Geometry check sheet. Reference: the model listing, model coordinates, mm. A direction names the side the tool comes from. Coordinates: 2 decimals unless noted, no trailing zeros. Loops run counter-clockwise (first coordinate to the right, second up) from the corner with the lowest first, then second, coordinate; pieces in that order, holes last.
from build123d import *

# Parameters (mm, degrees)
SKETCH1_R           = 1.617686351
BOSS_EXTRUDE1_DEPTH = 3.175
CUT_EXTRUDE1_DEPTH  = 1.5875


with BuildPart() as part:
    # Sketch1 → Boss-Extrude1 (new body)
    with BuildSketch(Plane.XY):
        with BuildLine():
            Line((2.376512113, 27.65079512), (87.842998078, 27.65079512))
            ThreePointArc((87.842998078, 27.65079512), (95.027202975, 24.675000017), (98.002998078, 17.49079512))
            Line((98.002998078, 17.49079512), (98.002998078, 7.726780525))
            ThreePointArc((98.002998078, 7.726780525), (95.027202975, 0.542575628), (87.842998078, -2.433219475))
            Line((87.842998078, -2.433219475), (2.376512113, -2.433219475))
            ThreePointArc((2.376512113, -2.433219475), (-4.807692784, 0.542575628), (-7.783487887, 7.726780525))
            Line((-7.783487887, 7.726780525), (-7.783487887, 17.49079512))
            ThreePointArc((-7.783487887, 17.49079512), (-4.807692784, 24.675000017), (2.376512113, 27.65079512))
        make_face()
        with Locations((-4.068268159, 12.608787822)):
            Circle(SKETCH1_R, mode=Mode.SUBTRACT)
    extrude(amount=BOSS_EXTRUDE1_DEPTH)

    # Sketch2 → Cut-Extrude1 (cut)
    # profile 1 of 3: a face of its own
    with BuildSketch(Plane.XY.offset(3.175)):
        with BuildLine():
            add(Edge.make_bspline(
                [(26.055314757, 25.363302374), (26.281041178, 25.357148606), (26.720344033, 25.345172305), (27.358603179, 25.255576736), (27.954181106, 25.10565776), (28.506593472, 24.887414053), (29.01635882, 24.61026015), (29.483989025, 24.268912351), (29.909556765, 23.870244327), (30.286214231, 23.412653315), (30.607890769, 22.914633219), (30.869796512, 22.384371241), (31.05896534, 21.825349006), (31.177064683, 21.240476881), (31.238829311, 20.630578255), (31.216595671, 19.996303633), (31.140690223, 19.333888525), (31.036825384, 18.891448023), (30.983281734, 18.663364293)],
                knots=[0, 0, 0, 0, 1.104647112, 2.14983532, 3.14775057, 4.103991838, 5.04949864, 5.980264506, 6.930364641, 7.896350518, 8.873894228, 9.826455567, 10.784034957, 11.753687545, 12.741876869, 13.777217861, 14.854127416, 16, 16, 16, 16], degree=3))
            Line((30.983281734, 18.663364293), (24.823323013, 14.893993808))
            add(Edge.make_bspline(
                [(24.823323013, 14.893993808), (24.913627964, 14.852436986), (25.056727556, 14.786584956), (25.204086092, 14.731009487), (25.258452012, 14.710505676)],
                knots=[0, 0, 0, 0, 1.262127295, 2, 2, 2, 2], degree=3))
            add(Edge.make_bspline(
                [(25.258452012, 14.710505676), (25.408658011, 14.633015541), (25.70455598, 14.480364025), (26.115294044, 14.203511612), (26.494533839, 13.898795938), (26.842207753, 13.563435468), (27.152694985, 13.192982522), (27.431219321, 12.792771569), (27.67927879, 12.362334709), (27.886089668, 11.901078686), (28.060682724, 11.422012006), (28.186061, 10.924600148), (28.269482345, 10.415995768), (28.312768514, 9.893514579), (28.306836135, 9.356553203), (28.251637963, 8.806740636), (28.160254496, 8.243184587), (28.061167889, 7.870056205), (28.010773994, 7.680288958)],
                knots=[0, 0, 0, 0, 0.984435104, 1.939285714, 2.881007598, 3.817426453, 4.749903878, 5.693661681, 6.656357472, 7.640950646, 8.636494269, 9.624663586, 10.626026113, 11.637696297, 12.67668649, 13.751023199, 14.856205644, 16, 16, 16, 16], degree=3))
            add(Edge.make_bspline(
                [(28.010773994, 7.680288958), (27.934336699, 7.418635325), (27.781985703, 6.897120378), (27.483880814, 6.140182715), (27.111873403, 5.418274722), (26.680602198, 4.723985098), (26.188457087, 4.059016869), (25.632410614, 3.42464569), (25.013362966, 2.8218799), (24.336555177, 2.259555831), (23.632617641, 1.73501911), (22.90194296, 1.286167719), (22.165575056, 0.899844078), (21.419750266, 0.582322921), (20.662474561, 0.341850589), (19.896429331, 0.167011128), (19.120780451, 0.059173369), (18.599040207, 0.044186513), (18.338328173, 0.036697626)],
                knots=[0, 0, 0, 0, 0.992207688, 1.977618791, 2.956517026, 3.945270844, 4.9506118, 5.965172583, 7.01356654, 8.093011568, 9.167098768, 10.207118156, 11.211733991, 12.192594754, 13.154449955, 14.10064625, 15.050898635, 16, 16, 16, 16], degree=3))
            Line((18.338328173, 0.036697626), (-1.667120743, 0.036697626))
            Line((-1.667120743, 0.036697626), (5.148152735, 25.363302374))
            Line((5.148152735, 25.363302374), (26.055314757, 25.363302374))
        make_face()
        Polygon((20.472033024, 6.196656347), (22.396037152, 13.373663571), (16.304231166, 9.567595459), (10.872982456, 9.567595459), (7.428648091, 6.196656347), align=None, mode=Mode.SUBTRACT)
        Polygon((22.867863777, 15.108937049), (23.953065015, 19.203343653), (10.652796698, 19.203343653), (7.648833849, 8.010567595), (14.820598555, 15.108937049), align=None, mode=Mode.SUBTRACT)
    # profile 2 of 3: a face of its own
    with BuildSketch(Plane.XY.offset(3.175)):
        with BuildLine():
            Line((40.052837977, 19.203343653), (39.654406605, 18.804912281))
            Line((39.654406605, 18.804912281), (37.515459236, 10.799587203))
            Line((37.515459236, 10.799587203), (43.712115583, 16.959545924))
            Line((43.712115583, 16.959545924), (54.511702786, 16.959545924))
            Line((54.511702786, 16.959545924), (53.028070175, 11.412961816))
            Line((53.028070175, 11.412961816), (39.80119711, 11.412961816))
            Line((39.80119711, 11.412961816), (36.902084623, 8.550546956))
            Line((36.902084623, 8.550546956), (36.283467492, 6.196656347))
            Line((36.283467492, 6.196656347), (51.28755418, 6.196656347))
            Line((51.28755418, 6.196656347), (55.817089783, 10.689494324))
            Line((55.817089783, 10.689494324), (56.828895769, 10.107574819))
            Line((56.828895769, 10.107574819), (48.278348813, 1.59372549))
            add(Edge.make_bspline(
                [(48.278348813, 1.59372549), (48.146238635, 1.46854593), (47.88717571, 1.223073677), (47.463918948, 0.909946193), (47.033190065, 0.640669228), (46.59089137, 0.416443393), (46.132411822, 0.249897844), (45.663767632, 0.128735888), (45.18249618, 0.052398669), (44.857011314, 0.041969808), (44.69246646, 0.036697626)],
                knots=[0, 0, 0, 0, 1.087710149, 2.132957327, 3.142311131, 4.123953504, 5.092881289, 6.053713067, 7.016078678, 8, 8, 8, 8], degree=3))
            Line((44.69246646, 0.036697626), (32.010815273, 0.036697626))
            add(Edge.make_bspline(
                [(32.010815273, 0.036697626), (31.858553331, 0.040498566), (31.561404624, 0.047916336), (31.12901049, 0.112299235), (30.724143119, 0.215813593), (30.34795697, 0.362171558), (30.00473747, 0.556447691), (29.68026271, 0.779177165), (29.39172657, 1.055755752), (29.136150439, 1.370039707), (28.916823334, 1.712741424), (28.744197554, 2.078286326), (28.60860469, 2.456433819), (28.533199597, 2.856014145), (28.494863315, 3.270534693), (28.507441143, 3.702944694), (28.564324089, 4.151146712), (28.63851974, 4.4497704), (28.676573787, 4.602930857)],
                knots=[0, 0, 0, 0, 1.094945795, 2.136855229, 3.137044923, 4.096584279, 5.030749513, 5.969051044, 6.920650617, 7.894578144, 8.878114772, 9.839711021, 10.797931648, 11.759527897, 12.756631189, 13.787866602, 14.865423694, 16, 16, 16, 16], degree=3))
            Line((28.676573787, 4.602930857), (30.018658411, 9.640990712))
            add(Edge.make_bspline(
                [(30.018658411, 9.640990712), (30.105903319, 9.92074967), (30.280853255, 10.481743003), (30.707081382, 11.263251403), (31.216779073, 12.016946207), (31.645281289, 12.457007159), (31.864024768, 12.681651187)],
                knots=[0, 0, 0, 0, 0.975136166, 1.955415087, 2.956272335, 4, 4, 4, 4], degree=3))
            Line((31.864024768, 12.681651187), (42.553519092, 23.26629515))
            add(Edge.make_bspline(
                [(42.553519092, 23.26629515), (42.728913539, 23.433821304), (43.070994593, 23.760556411), (43.621916797, 24.186341546), (44.183374604, 24.554272478), (44.766535305, 24.843767238), (45.358833813, 25.082449973), (45.970393028, 25.241335998), (46.595330871, 25.346832444), (47.017966502, 25.357802691), (47.229845201, 25.363302374)],
                knots=[0, 0, 0, 0, 1.104987577, 2.155115633, 3.169368792, 4.159784375, 5.118388166, 6.074904324, 7.034897349, 8, 8, 8, 8], degree=3))
            Line((47.229845201, 25.363302374), (61.903653251, 25.363302374))
            Line((61.903653251, 25.363302374), (60.236532508, 19.203343653))
            Line((60.236532508, 19.203343653), (40.052837977, 19.203343653))
        make_face()
    # profile 3 of 3: a face of its own
    with BuildSketch(Plane.XY.offset(3.175)):
        with BuildLine():
            Line((76.01126935, 25.363302374), (90.941960784, 25.363302374))
            Line((90.941960784, 25.363302374), (84.016594427, 0.036697626))
            Line((84.016594427, 0.036697626), (76.844829721, 0.036697626))
            Line((76.844829721, 0.036697626), (78.726893705, 6.956821465))
            Line((78.726893705, 6.956821465), (68.184189886, 6.956821465))
            Line((68.184189886, 6.956821465), (64.378121775, 3.18745098))
            Line((64.378121775, 3.18745098), (63.544561404, 0.036697626))
            Line((63.544561404, 0.036697626), (56.372796698, 0.036697626))
            Line((56.372796698, 0.036697626), (58.68998968, 8.660639835))
            add(Edge.make_bspline(
                [(58.68998968, 8.660639835), (58.755206826, 8.881790357), (58.885530435, 9.32371608), (59.134167271, 9.97030979), (59.42672045, 10.600153997), (59.771647631, 11.211465097), (60.158176901, 11.807063633), (60.588878909, 12.38650539), (61.069376559, 12.943271893), (61.414284452, 13.298477026), (61.589102167, 13.478513932)],
                knots=[0, 0, 0, 0, 0.972188851, 1.942727767, 2.918792729, 3.89888478, 4.900660299, 5.911935627, 6.941657613, 8, 8, 8, 8], degree=3))
            Line((61.589102167, 13.478513932), (71.591826625, 23.407843137))
            add(Edge.make_bspline(
                [(71.591826625, 23.407843137), (71.757107834, 23.56270533), (72.081611644, 23.866753032), (72.601980127, 24.266531398), (73.138947216, 24.602237151), (73.684800305, 24.883050108), (74.246444332, 25.101729813), (74.823529255, 25.252414119), (75.414191387, 25.344058862), (75.811733587, 25.35687144), (76.01126935, 25.363302374)],
                knots=[0, 0, 0, 0, 1.09520327, 2.15026038, 3.168190723, 4.15492977, 5.115689715, 6.0773418, 7.034972711, 8, 8, 8, 8], degree=3))
        make_face()
        with BuildLine():
            Line((80.179071207, 12.466707946), (81.987739938, 19.203343653))
            Line((81.987739938, 19.203343653), (68.981052632, 19.203343653))
            Line((68.981052632, 19.203343653), (68.582621259, 18.804912281))
            Line((68.582621259, 18.804912281), (64.996738906, 5.399793602))
            Line((64.996738906, 5.399793602), (70.826418989, 11.161320949))
            add(Edge.make_bspline(
                [(70.826418989, 11.161320949), (70.934905254, 11.264494776), (71.148060273, 11.467211858), (71.489484319, 11.734822191), (71.842666884, 11.964098761), (72.208262313, 12.144359196), (72.580718442, 12.291666427), (72.965176253, 12.387949636), (73.359703622, 12.455328131), (73.6273836, 12.462895723), (73.762229102, 12.466707946)],
                knots=[0, 0, 0, 0, 1.088018936, 2.137751703, 3.149265309, 4.143636785, 5.096896491, 6.055307392, 7.020348651, 8, 8, 8, 8], degree=3))
            Line((73.762229102, 12.466707946), (80.179071207, 12.466707946))
        make_face(mode=Mode.SUBTRACT)
    extrude(amount=-CUT_EXTRUDE1_DEPTH, mode=Mode.SUBTRACT)


solid = part.part
(1) Sectioned sample at A-A on x = 89. Record the cut outline in (y, z) (1 decimal), and give its area (3 significant figures).
Findings:
outline: (-2.4, 0) - (27.6, 0) - (27.6, 3.2) - (25.4, 3.2) - (25.4, 1.6) - (18.3, 1.6) - (18.3, 3.2) - (-2.4, 3.2) - close
area: 83.8 mm2
(2) Sectioned sample at B-B on z = 2.35. State how many separate pieces and enclosed holes the cut face has, and give its area (3 significant figures).
Findings:
separate pieces: 4
enclosed holes: 4
area: 1,720 mm2
(3) Access from +Z, -Z, +X, -X, +Y, -Y to the whole of each face (thin tool, end or side, straight path). Record for faces 4 (the flat face through (52.613, 5.91, 2.392)), 5 (the flat face through (17, 8, 3.175)).
Findings:
face 4: +Z
face 5: +Z, +X, -X, +Y, -Y
(4) Scan lines: L1, parallel to Y at x = 18, z = 1.8; L2, parallel to Y at x = 41.5, z = 1.7; L3, parallel to X at y = 5, z = 2. Record each from-to range of solid material in increasing order.
Findings:
L1: y = -2.43 to 0.04, 6.2 to 10.63, 15.11 to 19.2, 25.36 to 27.65
L2: y = -2.43 to 0.04, 6.2 to 11.41, 14.76 to 19.2, 22.22 to 27.65
L3: x = -7.41 to -0.33, 26.85 to 28.78, 51.7 to 57.71, 66.21 to 78.19, 85.37 to 97.63
(5) Gauge pin test, flat ends, axial feed: pin 1 Ø4 at (x, y) = (84, 7) entering from +Z (3 decimals); pin 2 Ø4 at (x, y) = (18, 21.5) entering from +Z. Record the tip position at first contact, or that the pin passes through.
Findings:
pin 1: stops at z = 3.175
pin 2: stops at z = 1.59
(6) Draft check along Y on faces 1 (the cylindrical face through (-4.728, 0.464, 1.565)), 2 (the flat face through (40.57, 13.836, 2.392)), 3 (the flat face through (45, 27.651, 2)). Enter one of: +Y half, -Y half, draft (parallel to the pull), parting line (faces both ways), or undercut.
Findings:
face 1: -Y half
face 2: undercut
face 3: +Y half
